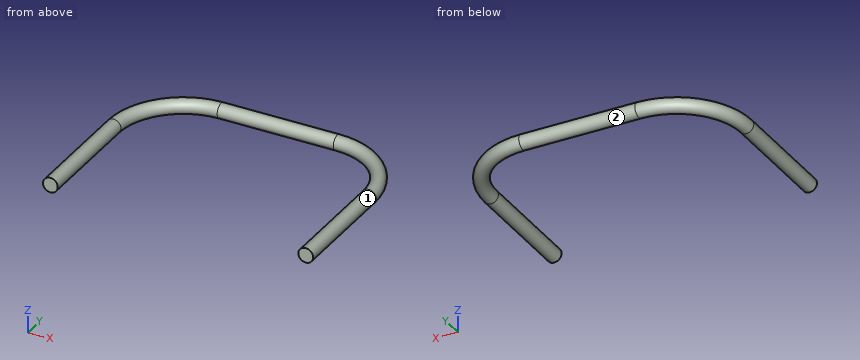
```python
from build123d import *

# Parameters (mm, degrees)
BALAYAGE1_PROFILE_R = 15.875


with BuildPart() as part:
    # Balayage1: sweep along a path in Esquisse2
    with BuildLine(Plane.XY) as balayage1_path:
        Line((0, 0), (0, 250))
        ThreePointArc((0, 250), (43.933982822, 356.066017178), (150, 400))
        Line((150, 400), (400, 400))
        ThreePointArc((400, 400), (506.066017178, 356.066017178), (550, 250))
        Line((550, 250), (550, 0))
    # Balayage1 profile (on start of the path) → Balayage1 (sweep)
    with BuildSketch(Plane.ZX):
        Circle(BALAYAGE1_PROFILE_R)
    sweep(path=balayage1_path.line)


solid = part.part
```
Could you check a few things on this model? Use its own coordinates, in mm. Face numbers are marked on the shaded views. A direction names the side the tool comes from. Coordinates: 2 decimals unless noted, no trailing zeros. Order: outer loops, then holes, each group sorted by start corner. A loop starts at its lowest first (then second) coordinate and runs counter-clockwise, first axis right, second up. Notation, with made-up numbers: M 39,23 L 91,23 A33 cw 91,61 Z; hole C 31,72.5 d6. An arc over 180 degrees is marked long. Use a Markdown table: item, result. Add a question column.
Q1. I want a section at C-C on x = 326.5. List the corners of the cut face in (y, z) for me (3 decimals).
Q2. Which directions (+Z, -Z, +X, -X, +Y, -Y) give clear straight access to the entire face, cutting with the end or side of a thin tool? Please do the marked faces 1 and 2.
Q3. I'm going to push flat-ended pins straight in: pin 1 (10 mm diameter, centred on x = 378.5, z = -9.5, fed in from +Y); pin 2 (4 mm diameter, centred on y = 310, z = -3.5, fed in from +X); pin 3 (5 mm diameter, centred on y = 309, z = 5.5, fed in from -X). Where does each tip first touch, or does it pass through?
Q4. I want a section at A-A on y = 105. List the corners of the cut face in (x, z) for me (3 decimals), then the cut area to 3 significant figures.
Q5. If I drill on L1, parallel to X at y = 91, z = 1; L2, parallel to X at y = 210, z = -13; L3, parallel to Y at x = 291, z = 2, over which ranges is the centre line in solid material (lowest first)?
Q6. I want a section at B-B on z = 0. List the corners of the cut face in (x, y) for me (3 decimals).
Checked values:
| question | item | result |
|---|---|---|
| 1 | outline | C 400,0 d31.75 |
| 2 | face 1 | -Y |
| 2 | face 2 | none |
| 3 | pin 1 | y = 415.22 |
| 3 | pin 2 | x = 555.1 |
| 3 | pin 3 | x = -5.23 |
| 4 | outline | C 0,0 d31.75; C 550,0 d31.75 |
| 4 | area | 1,580 mm² |
| 5 | L1 | -15.84 to 15.84, 534.16 to 565.84 |
| 5 | L2 | -9.11 to 9.11, 540.89 to 559.11 |
| 5 | L3 | 384.25 to 415.75 |
| 6 | outline | M -15.875,0 L 15.875,0 L 15.875,250 A134.125 cw 150,384.125 L 400,384.125 A134.125 cw 534.125,250 L 534.125,0 L 565.875,0 L 565.875,250 A165.875 ccw 400,415.875 L 150,415.875 A165.875 ccw -15.875,250 Z |
